The figure shows three views and two pictorial views of one solid part (mm, origin at its lowest corner). Answer the questions. Coordinates: 2 decimals unless noted, no trailing zeros. Order: outer loops, then holes, each group sorted by start corner. A loop starts at its lowest first (then second) coordinate and runs counter-clockwise, first axis right, second up. Notation, with made-up numbers: (-14.5, 37.5) - (8.5, 37.5) arc R11 ccw to (8.5, 42.5) - close; hole circle Ø8 at (72, 35.25). An arc over 180 degrees is marked (long way). Answer as a JSON object with one key per item and string values. Group by question number.
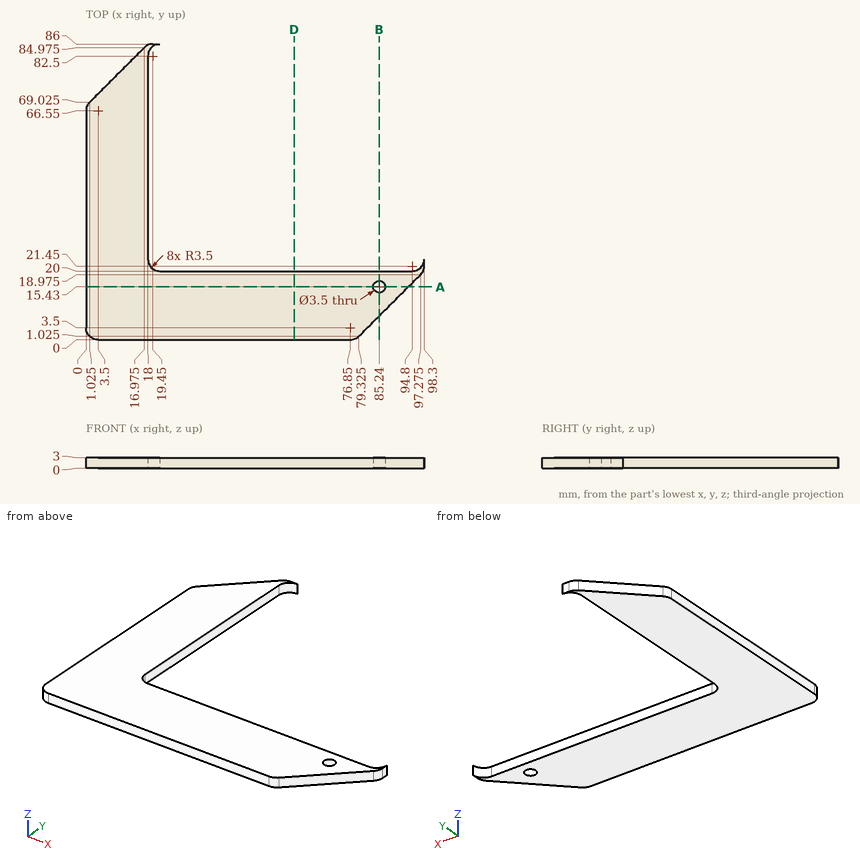
1. A cutting plane is placed at A-A on y = 15.43. Write down the section's boundary in (x, z), and give its area (3 significant figures).
2. A cutting plane is placed at D-D on x = 60.5. Write down the section's boundary in (y, z), and give its area (3 significant figures).
3. A cutting plane is placed at B-B on x = 85.24. Write down the section's boundary in (y, z), and give its area (3 significant figures).
4. Given pin 1 (2 mm diameter, centred on x = 85.24, y = 15.43, fed in from +Z); pin 2 (0.9 mm diameter, centred on y = 67, z = 2, fed in from +X), each flat-ended and moving along its own axis, determine where each tip first touches the part or whether it passes through.
5. Straight lines are drawn through the part: L1, parallel to Y at x = 25.5, z = 1.55; L2, parallel to Y at x = 85.24, z = 2.2; L3, parallel to Y at x = 85.5, z = 2.35. For each, find the intervals that lie inside material, in ascending order.
Derived:
{
 "1": {"outline": "(0, 0) - (83.49, 0) - (83.49, 3) - (0, 3) - close; (86.99, 0) - (93.73, 0) - (93.73, 3) - (86.99, 3) - close", "area": "271 mm2"},
 "2": {"outline": "(0, 0) - (20, 0) - (20, 3) - (0, 3) - close", "area": "60.0 mm2"},
 "3": {"outline": "(6.94, 0) - (13.68, 0) - (13.68, 3) - (6.94, 3) - close; (17.18, 0) - (20, 0) - (20, 3) - (17.18, 3) - close", "area": "28.7 mm2"},
 "4": {"pin 1": "passes through", "pin 2": "stops at x = 18"},
 "5": {"L1": "y = 0 to 20", "L2": "y = 6.94 to 13.68, 17.18 to 20", "L3": "y = 7.2 to 13.7, 17.16 to 20"}
}
